Autodesk Inventor part; units mm, degrees
ref_plane "YZ Plane" through (0, 0, 0) normal (1, 0, 0) x (0, 1, 0)
ref_plane "XZ Plane" through (0, 0, 0) normal (0, 1, 0) x (-1, 0, 0)
ref_plane "XY Plane" through (0, 0, 0) normal (0, 0, 1) x (1, 0, 0)
sketch "スケッチ1" plane through (0, 0, 0) normal (0, 1, 0) x (-1, 0, 0)
  line L0 (130, 1.5) -> (-130, 1.5)
  line L1 (-130, 1.5) -> (-130, -1.5)
  line L2 (-130, -1.5) -> (130, -1.5)
  line L3 (130, -1.5) -> (130, 1.5)
  line L4 (130, 1.5) -> (-130, -1.5) construction
  line L5 (-130, 1.5) -> (130, -1.5) construction
  point P0 (0, 0)
  dimension "d0" = 260
  dimension "d1" = 3
extrude "押し出し1" add sketch "スケッチ1" along normal blind 120
sketch "スケッチ3" plane through (-130, 0, 1.5) normal (0, 0, 1) x (1, 0, 0)
  circle A0 centre (60, 60) radius 12.5
  circle A1 centre (130, 60) radius 12.5
  circle A2 centre (200, 60) radius 12.5
  line L0 (0, 0) -> (0, 120)
  line L1 (260, 0) -> (260, 120)
  point P0 (130, 0)
  point P1 (0, 60)
  point P2 (260, 60)
  dimension "d10" = 25
  dimension "d11" = 25
  dimension "d12" = 25
  dimension "d15" = 60
  dimension "d16" = 60
  dimension "d18" = 0
  dimension "d21" = 0
  dimension "d71" = 0
  dimension "d72" = 70
extrude "押し出し3" cut sketch "スケッチ3" against normal through all
sketch "スケッチ5" plane through (130, 0, -1.5) normal (0, 0, -1) x (-1, 0, 0)
  line L0 (0, 0) -> (260, 0)
  line L1 (0, 120) -> (3, 120)
  line L2 (3, 120) -> (3, 0)
  line L3 (3, 0) -> (0, 0)
  line L4 (0, 0) -> (0, 120)
  line L5 (0, 105) -> (3, 105)
  line L6 (3, 105) -> (3, 15)
  line L7 (3, 15) -> (0, 15)
  line L8 (0, 15) -> (0, 105)
  line L9 (0, 120) -> (260, 120)
  line L10 (130, 120) -> (130, 0)
  line L11 (260, 0) -> (0, 0)
  line L12 (260, 120) -> (257, 120)
  line L13 (257, 120) -> (257, 0)
  line L14 (260, 0) -> (260, 120)
  line L15 (260, 105) -> (257, 105)
  line L16 (257, 15) -> (260, 15)
  point P0 (1.5, 105)
  point P1 (1.5, 120)
  point P2 (1.5, 15)
  point P3 (1.5, 0)
  point P4 (258.5, 15)
  point P5 (257, 0)
  point P6 (257, 120)
  point P7 (0, 15)
  point P8 (3, 105)
  dimension "d22" = 3
  dimension "d23" = 15
  dimension "d24" = 15
extrude "押し出し4" cut sketch "スケッチ5" against normal through all contours L4 L7 L2 L0 | L4 L5 L2 L7 | L4 L1 L2 L5 | L13 L16 L14 L0 | L13 L15 L14 L16 | L9 L14 L15 L13
sketch "スケッチ8" plane through (-127, 0, 1.5) normal (0, 0, 1) x (1, 0, 0)
  circle A0 centre (20, 100) radius 1.6
  circle A1 centre (20, 20) radius 1.6
  line L0 (0, 120) -> (0, 0)
  line L1 (0, 120) -> (254, 120)
  line L2 (0, 0) -> (254, 0)
  line L3 (127, 120) -> (127, 0)
  circle A2 centre (234, 100) radius 1.6
  circle A3 centre (234, 20) radius 1.6
  circle A4 centre (20, 60) radius 1.6
  circle A5 centre (234, 60) radius 1.6
  dimension "d31" = 20
  dimension "d32" = 20
  dimension "d33" = 20
  dimension "d34" = 20
  dimension "d35" = 3.2
  dimension "d36" = 3.2
  dimension "d73" = 3.2
  dimension "d74" = 40
  dimension "d75" = 20
extrude "押し出し7" cut sketch "スケッチ8" against normal through all contours A0 | A1 | A2 | A3 | A4 | A5
fillet "フィレット1" radius 5 4 edges at (-127, 120, 0) (-127, 0, 0) (127, 120, 0) (127, 0, 0)
sketch "スケッチ13" plane through (-122, 0, 1.5) normal (0, 0, 1) x (1, 0, 0)
  line L0 (244, 120) -> (0, 120)
  line L1 (122, 120) -> (122, 0)
  circle A0 centre (15, 110) radius 1.6
  circle A1 centre (15, 10) radius 1.6
  circle A2 centre (15, 60) radius 1.6
  circle A3 centre (122, 60) radius 12.5
  line L2 (122, 60) -> (122, 88.3789)
  point P0 (26, 80)
  point P1 (26, 40)
  point P2 (218, 80)
  point P3 (218, 40)
  dimension "d76" = 11
  dimension "d77" = 40
  dimension "d78" = 20
  dimension "d79" = 11
hole "穴1" at (-96, 80, 1.5) at (-96, 40, 1.5) at (96, 40, 1.5) at (96, 80, 1.5) direction (0, 0, -1) diameter 3.2 end through all
equation "\"d36\" = d35"
equation "\"d73\" = d35"
properties part number "BP_BOX-Front-120" material "アセタール樹脂、白"
The model under review builds one solid part; all positions refer to its coordinate system, in mm. Give positions to 0.01 mm unless a question says otherwise; leave off trailing zeros. Write each loop counter-clockwise with the first axis right and the second up, starting at its lowest first coordinate (ties: lowest second). Pieces come first, ordered by that corner, then holes. Notation, with made-up numbers: (80.5, 67.25) - (97.5, 67.25) arc R13 cw to (97.5, 76.25) - close; hole circle Ø6 at (-15, -24). An arc over 180 degrees is marked (long way). Answer in a Markdown table with one row per item. Add a question column.
1. Draft analysis for pull direction Y (two halves, no side actions). For faces 1 (the cylindrical face through (-71.627, 72.394, 0.021)), 2 (the cylindrical face through (126, 118, 0)), 3 (the cylindrical face through (-126, 2, 0)), state which applies: +Y half, -Y half, draft (parallel to the pull), parting line (faces both ways), or undercut.
2. We need section A-A on x = 70. Write out the cut boundary in (y, z).
3. Wall thickness on line 1 along X through (y, z) = (100, -0.75); line 2 along X through (y, z) = (64.5, 0.85); line 3 along Y through (x, z) = (-70, -0.35): over which ranges is each line inside the solid? List them lowest first. Write a range as [from, to].
4. Insertion check: P1, Ø5, axis at x = 96, y = 40, coming from the +Z side; P2, Ø3, axis at x = -107, y = 20, coming from the +Z side. Each pin has a flat end and moves straight along its axis. Give the tip position at first contact, or say it passes through.
5. We need section C-C on x = -1. Write out the cut boundary in (y, z).
6. We need section B-B on z = -0.25. State how many separate pieces and enclosed holes the cut face has, then the cut area to 3 significant figures.
Ans:
| question | item | result |
|---|---|---|
| 1 | face 1 | undercut |
| 1 | face 2 | +Y half |
| 1 | face 3 | -Y half |
| 2 | outline | (0, -1.5) - (47.5, -1.5) - (47.5, 1.5) - (0, 1.5) - close; (72.5, -1.5) - (120, -1.5) - (120, 1.5) - (72.5, 1.5) - close |
| 3 | line 1 | x = [-127, -108.6], [-105.4, 105.4], [108.6, 127] |
| 3 | line 2 | x = [-127, -81.66], [-58.34, -11.66], [11.66, 58.34], [81.66, 127] |
| 3 | line 3 | y = [0, 47.5], [72.5, 120] |
| 4 | P1 | stops at z = 1.5 |
| 4 | P2 | passes through |
| 5 | outline | (0, -1.5) - (47.54, -1.5) - (47.54, 1.5) - (0, 1.5) - close; (72.46, -1.5) - (120, -1.5) - (120, 1.5) - (72.46, 1.5) - close |
| 6 | separate pieces | 1 |
| 6 | enclosed holes | 13 |
| 6 | area | 28,900 mm^2 |
